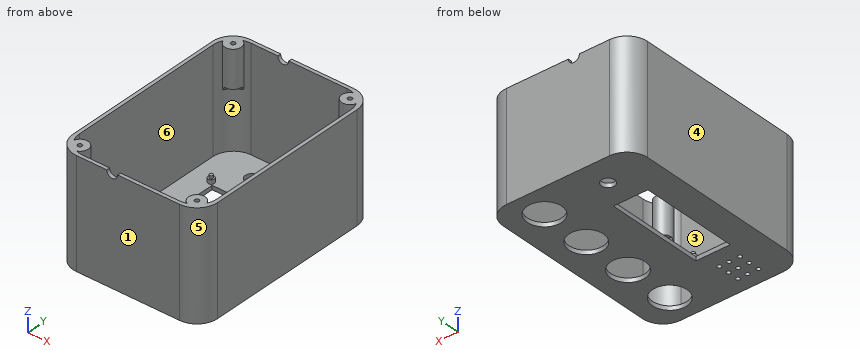
from build123d import *

# Parameters (mm, degrees)
CYLINDER029_R          = 12.5
CYLINDER029_DEPTH      = 10
ARRAY005_Y_COUNT       = 4
ARRAY005_Y_PITCH       = 36
CYLINDER028_R          = 14
CYLINDER028_DEPTH      = 3
ARRAY004_Y_COUNT       = 4
ARRAY004_Y_PITCH       = 36
CYLINDER027_R          = 4.8
CYLINDER027_DEPTH      = 10
CYLINDER026_W          = 4
CYLINDER026_H          = 157
CYLINDER026_ANGLE      = 180
CYLINDER026_ROLL_ANGLE = -90
CYLINDER023_R          = 1.5
CYLINDER023_DEPTH      = 10
CYLINDER024_R          = 1.5
CYLINDER024_DEPTH      = 10
CYLINDER018_R          = 1.5
CYLINDER018_DEPTH      = 10
CYLINDER020_R          = 1.5
CYLINDER020_DEPTH      = 10
CYLINDER021_R          = 1.5
CYLINDER021_DEPTH      = 10
CYLINDER025_R          = 1.5
CYLINDER025_DEPTH      = 10
CYLINDER019_R          = 1.5
CYLINDER019_DEPTH      = 10
CYLINDER022_R          = 1.5
CYLINDER022_DEPTH      = 10
CYLINDER017_R          = 1.5
CYLINDER017_DEPTH      = 10
CYLINDER008_R          = 1.6
CYLINDER008_DEPTH      = 28
CYLINDER010_R          = 1.6
CYLINDER010_DEPTH      = 27
CYLINDER009_R          = 1.6
CYLINDER009_DEPTH      = 28
CYLINDER011_R          = 1.6
CYLINDER011_DEPTH      = 29
CYLINDER005_R          = 6
CYLINDER005_DEPTH      = 27
CYLINDER007_R          = 6
CYLINDER007_DEPTH      = 27
CYLINDER004_R          = 6
CYLINDER004_DEPTH      = 27
CYLINDER003_R          = 6
CYLINDER003_DEPTH      = 27
CYLINDER002_R          = 2.3
CYLINDER002_DEPTH      = 3
ARRAY002_X_COUNT       = 2
ARRAY002_X_PITCH       = 31
ARRAY002_Y_COUNT       = 2
ARRAY002_Y_PITCH       = 75.2
CYLINDER001_R          = 1.3
CYLINDER001_DEPTH      = 5
ARRAY001_X_COUNT       = 2
ARRAY001_X_PITCH       = 31
ARRAY001_Y_COUNT       = 2
ARRAY001_Y_PITCH       = 75.2
BOX002_W               = 25
BOX002_H               = 71
BOX002_DEPTH           = 10
CYLINDER_R             = 14
CYLINDER_DEPTH         = 10
ARRAY_Y_COUNT          = 4
ARRAY_Y_PITCH          = 36
BOX001_W               = 100
BOX001_H               = 145
BOX001_DEPTH           = 75
BOX_W                  = 105
BOX_H                  = 150
BOX_DEPTH              = 78
FILLET_R               = 15
FILLET001_R            = 15
CHAMFER_SIZE           = 6.3
CHAMFER002_SIZE        = 6
CHAMFER003_SIZE        = 6
CHAMFER004_SIZE        = 6


with BuildPart() as botones003:
    # Cylinder029 → Cylinder029 (new body)
    with BuildSketch(Plane(origin=(80, 25, 0), x_dir=(1, 0, 0), z_dir=(0, 0, 1))):
        Circle(CYLINDER029_R)
    extrude(amount=CYLINDER029_DEPTH)

    # Array005 Y: Botones003 ×4


with BuildPart() as botones003_1:
    add(botones003.part)
    with Locations(*[(0, i * ARRAY005_Y_PITCH, 0) for i in range(1, ARRAY005_Y_COUNT)]):
        add(botones003.part)


with BuildPart() as botones003_2:
    # Array005 placement: moved
    add(botones003_1.part.moved(Location((0, -4, -2))))


with BuildPart() as botones002:
    # Cylinder028 → Cylinder028 (new body)
    with BuildSketch(Plane(origin=(80, 25, 0), x_dir=(1, 0, 0), z_dir=(0, 0, 1))):
        Circle(CYLINDER028_R)
    extrude(amount=CYLINDER028_DEPTH)

    # Array004 Y: Botones002 ×4


with BuildPart() as botones002_1:
    add(botones002.part)
    with Locations(*[(0, i * ARRAY004_Y_PITCH, 0) for i in range(1, ARRAY004_Y_COUNT)]):
        add(botones002.part)


with BuildPart() as botones002_2:
    # Array004 placement: moved
    add(botones002_1.part.moved(Location((0, -4, 0))))


with BuildPart() as cilindro027:
    # Cylinder027 → Cylinder027 (new body)
    with BuildSketch(Plane(origin=(33, 130, -5), x_dir=(1, 0, 0), z_dir=(0, 0, 1))):
        Circle(CYLINDER027_R)
    extrude(amount=CYLINDER027_DEPTH)


with BuildPart() as cilindro026:
    # Cylinder026 → Cylinder026 (revolve)
    with BuildSketch(Plane.XZ):
        with Locations((2, 78.5)):
            Rectangle(CYLINDER026_W, CYLINDER026_H)
    revolve(axis=Axis((0, 0, 0), (0, 0, 1)), revolution_arc=CYLINDER026_ANGLE)


with BuildPart() as cilindro026_1:
    # Cylinder026 roll: moved
    add(cilindro026.part.rotate(Axis((0, 0, 0), (1, 0, 0)), CYLINDER026_ROLL_ANGLE))


with BuildPart() as cilindro026_2:
    # Cylinder026 placement: moved
    add(cilindro026_1.part.moved(Location((41, -3, 78))))


with BuildPart() as cilindro023:
    # Cylinder023 → Cylinder023 (new body)
    with BuildSketch(Plane(origin=(39, 27, 0), x_dir=(1, 0, 0), z_dir=(0, 0, 1))):
        Circle(CYLINDER023_R)
    extrude(amount=CYLINDER023_DEPTH)


with BuildPart() as cilindro024:
    # Cylinder024 → Cylinder024 (new body)
    with BuildSketch(Plane(origin=(39, 19, 0), x_dir=(1, 0, 0), z_dir=(0, 0, 1))):
        Circle(CYLINDER024_R)
    extrude(amount=CYLINDER024_DEPTH)


with BuildPart() as cilindro018:
    # Cylinder018 → Cylinder018 (new body)
    with BuildSketch(Plane(origin=(24, 19, 0), x_dir=(1, 0, 0), z_dir=(0, 0, 1))):
        Circle(CYLINDER018_R)
    extrude(amount=CYLINDER018_DEPTH)


with BuildPart() as cilindro020:
    # Cylinder020 → Cylinder020 (new body)
    with BuildSketch(Plane(origin=(32, 27, 0), x_dir=(1, 0, 0), z_dir=(0, 0, 1))):
        Circle(CYLINDER020_R)
    extrude(amount=CYLINDER020_DEPTH)


with BuildPart() as cilindro021:
    # Cylinder021 → Cylinder021 (new body)
    with BuildSketch(Plane(origin=(32, 19, 0), x_dir=(1, 0, 0), z_dir=(0, 0, 1))):
        Circle(CYLINDER021_R)
    extrude(amount=CYLINDER021_DEPTH)


with BuildPart() as cilindro025:
    # Cylinder025 → Cylinder025 (new body)
    with BuildSketch(Plane(origin=(39, 11, 0), x_dir=(1, 0, 0), z_dir=(0, 0, 1))):
        Circle(CYLINDER025_R)
    extrude(amount=CYLINDER025_DEPTH)


with BuildPart() as cilindro019:
    # Cylinder019 → Cylinder019 (new body)
    with BuildSketch(Plane(origin=(24, 11, 0), x_dir=(1, 0, 0), z_dir=(0, 0, 1))):
        Circle(CYLINDER019_R)
    extrude(amount=CYLINDER019_DEPTH)


with BuildPart() as cilindro022:
    # Cylinder022 → Cylinder022 (new body)
    with BuildSketch(Plane(origin=(32, 11, 0), x_dir=(1, 0, 0), z_dir=(0, 0, 1))):
        Circle(CYLINDER022_R)
    extrude(amount=CYLINDER022_DEPTH)


with BuildPart() as obj1:
    # Cylinder017 → Cylinder017 (new body)
    with BuildSketch(Plane(origin=(24, 27, 0), x_dir=(1, 0, 0), z_dir=(0, 0, 1))):
        Circle(CYLINDER017_R)
    extrude(amount=CYLINDER017_DEPTH)

    # Fusion007: union Cilindro023, Cilindro024, Cilindro018, Cilindro020, Cilindro021, Cilindro025, Cilindro019, Cilindro022
    add(cilindro023.part)
    add(cilindro024.part)
    add(cilindro018.part)
    add(cilindro020.part)
    add(cilindro021.part)
    add(cilindro025.part)
    add(cilindro019.part)
    add(cilindro022.part)


with BuildPart() as cilindro008:
    # Cylinder008 → Cylinder008 (new body)
    with BuildSketch(Plane(origin=(10, 141, 51), x_dir=(1, 0, 0), z_dir=(0, 0, 1))):
        Circle(CYLINDER008_R)
    extrude(amount=CYLINDER008_DEPTH)


with BuildPart() as cilindro010:
    # Cylinder010 → Cylinder010 (new body)
    with BuildSketch(Plane(origin=(95, 141, 51), x_dir=(1, 0, 0), z_dir=(0, 0, 1))):
        Circle(CYLINDER010_R)
    extrude(amount=CYLINDER010_DEPTH)


with BuildPart() as cilindro009:
    # Cylinder009 → Cylinder009 (new body)
    with BuildSketch(Plane(origin=(95, 9, 51), x_dir=(1, 0, 0), z_dir=(0, 0, 1))):
        Circle(CYLINDER009_R)
    extrude(amount=CYLINDER009_DEPTH)


with BuildPart() as fusion005:
    # Cylinder011 → Cylinder011 (new body)
    with BuildSketch(Plane(origin=(10, 9, 51), x_dir=(1, 0, 0), z_dir=(0, 0, 1))):
        Circle(CYLINDER011_R)
    extrude(amount=CYLINDER011_DEPTH)

    # Fusion005: union Cilindro008, Cilindro010, Cilindro009
    add(cilindro008.part)
    add(cilindro010.part)
    add(cilindro009.part)


with BuildPart() as fusion005_1:
    # Fusion005 placement: moved
    add(fusion005.part.moved(Location((0, 0, 2))))


with BuildPart() as cilindro005:
    # Cylinder005 → Cylinder005 (new body)
    with BuildSketch(Plane(origin=(95, 141, 51), x_dir=(1, 0, 0), z_dir=(0, 0, 1))):
        Circle(CYLINDER005_R)
    extrude(amount=CYLINDER005_DEPTH)


with BuildPart() as cilindro007:
    # Cylinder007 → Cylinder007 (new body)
    with BuildSketch(Plane(origin=(10, 141, 51), x_dir=(1, 0, 0), z_dir=(0, 0, 1))):
        Circle(CYLINDER007_R)
    extrude(amount=CYLINDER007_DEPTH)


with BuildPart() as fusion003:
    # Cylinder004 → Cylinder004 (new body)
    with BuildSketch(Plane(origin=(95, 9, 51), x_dir=(1, 0, 0), z_dir=(0, 0, 1))):
        Circle(CYLINDER004_R)
    extrude(amount=CYLINDER004_DEPTH)

    # Fusion003: union Cilindro005, Cilindro007
    add(cilindro005.part)
    add(cilindro007.part)


with BuildPart() as cilindro003:
    # Cylinder003 → Cylinder003 (new body)
    with BuildSketch(Plane(origin=(10, 9, 51), x_dir=(1, 0, 0), z_dir=(0, 0, 1))):
        Circle(CYLINDER003_R)
    extrude(amount=CYLINDER003_DEPTH)


with BuildPart() as array002:
    # Cylinder002 → Cylinder002 (new body)
    with BuildSketch(Plane(origin=(18, 37.5, 3), x_dir=(1, 0, 0), z_dir=(0, 0, 1))):
        Circle(CYLINDER002_R)
    extrude(amount=CYLINDER002_DEPTH)

    # Array002 X: Array002 ×2


with BuildPart() as array002_1:
    add(array002.part)
    with Locations(*[(i * ARRAY002_X_PITCH, 0, 0) for i in range(1, ARRAY002_X_COUNT)]):
        add(array002.part)

    # Array002 Y: Array002 ×2


with BuildPart() as array002_2:
    add(array002_1.part)
    with Locations(*[(0, i * ARRAY002_Y_PITCH, 0) for i in range(1, ARRAY002_Y_COUNT)]):
        add(array002_1.part)


with BuildPart() as fusion:
    # Cylinder001 → Cylinder001 (new body)
    with BuildSketch(Plane(origin=(18, 37.5, 3), x_dir=(1, 0, 0), z_dir=(0, 0, 1))):
        Circle(CYLINDER001_R)
    extrude(amount=CYLINDER001_DEPTH)

    # Array001 X: Fusion ×2


with BuildPart() as fusion_1:
    add(fusion.part)
    with Locations(*[(i * ARRAY001_X_PITCH, 0, 0) for i in range(1, ARRAY001_X_COUNT)]):
        add(fusion.part)

    # Array001 Y: Fusion ×2


with BuildPart() as fusion_2:
    add(fusion_1.part)
    with Locations(*[(0, i * ARRAY001_Y_PITCH, 0) for i in range(1, ARRAY001_Y_COUNT)]):
        add(fusion_1.part)

    # Fusion: union Array002
    add(array002_2.part)


with BuildPart() as cubo002:
    # Box002 → Box002 (new body)
    with BuildSketch(Plane(origin=(20.5, 39.5, -1), x_dir=(1, 0, 0), z_dir=(0, 0, 1))):
        with Locations((12.5, 35.5)):
            Rectangle(BOX002_W, BOX002_H)
    extrude(amount=BOX002_DEPTH)


with BuildPart() as botones:
    # Cylinder → Cylinder (new body)
    with BuildSketch(Plane(origin=(80, 25, 0), x_dir=(1, 0, 0), z_dir=(0, 0, 1))):
        Circle(CYLINDER_R)
    extrude(amount=CYLINDER_DEPTH)

    # Array Y: Botones ×4


with BuildPart() as botones_1:
    add(botones.part)
    with Locations(*[(0, i * ARRAY_Y_PITCH, 0) for i in range(1, ARRAY_Y_COUNT)]):
        add(botones.part)


with BuildPart() as botones_2:
    # Array placement: moved
    add(botones_1.part.moved(Location((0, -4, -2))))


with BuildPart() as cubo001:
    # Box001 → Box001 (new body)
    with BuildSketch(Plane(origin=(2.5, 2.5, 3), x_dir=(1, 0, 0), z_dir=(0, 0, 1))):
        with Locations((50, 72.5)):
            Rectangle(BOX001_W, BOX001_H)
    extrude(amount=BOX001_DEPTH)


with BuildPart() as cut012:
    # Box → Box (new body)
    with BuildSketch(Plane.XY):
        with Locations((52.5, 75)):
            Rectangle(BOX_W, BOX_H)
    extrude(amount=BOX_DEPTH)

    # Cut: cut Cubo001
    add(cubo001.part, mode=Mode.SUBTRACT)

    # Cut001: cut Botones
    add(botones_2.part, mode=Mode.SUBTRACT)

    # Cut002: cut Cubo002
    add(cubo002.part, mode=Mode.SUBTRACT)

    # Fillet
    fillet_edges = [cut012.edges().sort_by_distance(p)[0] for p in [
        (2.5, 2.5, 40.5),
        (2.5, 147.5, 40.5),
        (102.5, 2.5, 40.5),
        (102.5, 147.5, 40.5),
    ]]
    fillet(fillet_edges, radius=FILLET_R)

    # Fillet001
    fillet001_edges = [cut012.edges().sort_by_distance(p)[0] for p in [
        (0, 0, 39),
        (0, 150, 39),
        (105, 150, 39),
        (105, 0, 39),
    ]]
    fillet(fillet001_edges, radius=FILLET001_R)

    # Fusion001: union Fusion
    add(fusion_2.part)

    # Fusion002: union Cilindro003
    add(cilindro003.part)

    # Chamfer
    chamfer_edges = [cut012.edges().sort_by_distance(p)[0] for p in [
        (7.575675, 6.252432, 51),
    ]]
    chamfer(chamfer_edges, length=CHAMFER_SIZE)

    # Fusion004: union Fusion003
    add(fusion003.part)

    # Chamfer002
    chamfer002_edges = [cut012.edges().sort_by_distance(p)[0] for p in [
        (7.575675, 143.747568, 51),
    ]]
    chamfer(chamfer002_edges, length=CHAMFER002_SIZE)

    # Chamfer003
    chamfer003_edges = [cut012.edges().sort_by_distance(p)[0] for p in [
        (97.424325, 143.747568, 51),
    ]]
    chamfer(chamfer003_edges, length=CHAMFER003_SIZE)

    # Chamfer004
    chamfer004_edges = [cut012.edges().sort_by_distance(p)[0] for p in [
        (97.424325, 6.252432, 51),
    ]]
    chamfer(chamfer004_edges, length=CHAMFER004_SIZE)

    # Cut003: cut Fusion005
    add(fusion005_1.part, mode=Mode.SUBTRACT)

    # Cut009: cut obj1
    add(obj1.part, mode=Mode.SUBTRACT)

    # Cut010: cut Cilindro026
    add(cilindro026_2.part, mode=Mode.SUBTRACT)

    # Cut011: cut Cilindro027
    add(cilindro027.part, mode=Mode.SUBTRACT)

    # Fusion011: union Botones002
    add(botones002_2.part)

    # Cut012: cut Botones003
    add(botones003_2.part, mode=Mode.SUBTRACT)


solid = cut012.part
Here's how the part is built. I have some questions about the finished solid (model axes, mm). Face numbers are marked on the shaded views. A direction names the side the tool comes from. Coordinates: 2 decimals unless noted, no trailing zeros. Order: outer loops, then holes, each group sorted by start corner. A loop starts at its lowest first (then second) coordinate and runs counter-clockwise, first axis right, second up. Notation, with made-up numbers: (74, 34.5) - (133, 34.5) arc R25 cw to (133, 53.5) - close; hole circle Ø9 at (66, 49.25). An arc over 180 degrees is marked (long way). Use CSV: the item, a comma, the result in double quotes. Start each with the question number.
1. Suppose I cut it at D-D on z = 72. List the corners of the cut face in (x, y) for me.
2. Suppose I cut it at C-C on z = 18. List the corners of the cut face in (x, y) for me.
3. If we mould it in two halves opening along Y, with no side actions, what happens to the marked faces 4, 5 and 6? For each: +Y half, -Y half, draft (parallel to the pull), parting line (faces both ways), or undercut.
4. Please list where these lines run through material, in increasing order: line 1 (Y direction, x = 80, z = 2.2); line 2 (Y direction, x = 61.5, z = 49); line 3 (X direction, y = 101.5, z = 59.5). Write a range as from..to.
5. I'm going to push flat-ended pins straight in: pin 1 (11 mm diameter, centred on x = 33, y = 130, fed in from +Z); pin 2 (1.4 mm diameter, centred on x = 49.5, y = 112, fed in from +Z); pin 3 (5 mm diameter, centred on x = 94.5, z = 41.5, fed in from -Y); pin 4 (4 mm diameter, centred on x = 70.5, y = 90.5, fed in from -Z). Where does each tip first touch, or does it pass through?
6. For the marked faces 1, 2 and 3, which set-ups out of +Z, -Z, +X, -X, +Y, -Y let a thin tool reach every point of the face, with its end or its side?
7. Suppose I cut it at B-B on y = 57. List the corners of the cut face in (x, z) for me, then the cut area to 3 significant figures.
8. Suppose I cut it at A-A on x = 72.5. List the corners of the cut face in (y, z) for me.
Output:
1,outline,"(0, 15) arc R15 ccw to (15, 0) - (90, 0) arc R15 ccw to (105, 15) - (105, 135) arc R15 ccw to (90, 150) - (15, 150) arc R15 ccw to (0, 135) - close; hole (2.5, 17.5) arc R15 ccw to (4.2, 10.55) arc R6 cw (long way) to (12.26, 3.44) arc R15 ccw to (17.5, 2.5) - (87.5, 2.5) arc R15 ccw to (92.74, 3.44) arc R6 cw (long way) to (100.8, 10.55) arc R15 ccw to (102.5, 17.5) - (102.5, 132.5) arc R15 ccw to (100.8, 139.45) arc R6 cw (long way) to (92.74, 146.56) arc R15 ccw to (87.5, 147.5) - (17.5, 147.5) arc R15 ccw to (12.26, 146.56) arc R6 cw (long way) to (4.2, 139.45) arc R15 ccw to (2.5, 132.5) - close; hole circle Ø3.2 at (10, 9); hole circle Ø3.2 at (10, 141); hole circle Ø3.2 at (95, 9); hole circle Ø3.2 at (95, 141)"
2,outline,"(0, 15) arc R15 ccw to (15, 0) - (90, 0) arc R15 ccw to (105, 15) - (105, 135) arc R15 ccw to (90, 150) - (15, 150) arc R15 ccw to (0, 135) - close; hole (2.5, 17.5) arc R15 ccw to (17.5, 2.5) - (87.5, 2.5) arc R15 ccw to (102.5, 17.5) - (102.5, 132.5) arc R15 ccw to (87.5, 147.5) - (17.5, 147.5) arc R15 ccw to (2.5, 132.5) - close"
3,face 4,"draft"
3,face 5,"-Y half"
3,face 6,"undercut"
4,line 1,"y = 0..8.5, 33.5..44.5, 69.5..80.5, 105.5..116.5, 141.5..150"
4,line 2,"y = 0..2.5, 147.5..150"
4,line 3,"x = 0..2.5, 102.5..105"
5,pin 1,"stops at z = 3"
5,pin 2,"stops at z = 8"
5,pin 3,"stops at y = 0.13"
5,pin 4,"passes through"
6,face 1,"+Z, -Z, +X, -X, -Y"
6,face 2,"none"
6,face 3,"+Z"
7,outline,"(0, 0) - (20.5, 0) - (20.5, 3) - (2.5, 3) - (2.5, 78) - (0, 78) - close; (45.5, 0) - (67.5, 0) - (67.5, 3) - (45.5, 3) - close; (92.5, 0) - (105, 0) - (105, 78) - (102.5, 78) - (102.5, 3) - (92.5, 3) - close"
7,area,"540 mm2"
8,outline,"(0, 0) - (11, 0) - (11, 3) - (2.5, 3) - (2.5, 78) - (0, 78) - close; (31, 0) - (47, 0) - (47, 3) - (31, 3) - close; (67, 0) - (83, 0) - (83, 3) - (67, 3) - close; (103, 0) - (119, 0) - (119, 3) - (103, 3) - close; (139, 0) - (150, 0) - (150, 78) - (147.5, 78) - (147.5, 3) - (139, 3) - close"
